Build history of the part. All positions in model axes, mm. Face numbers are marked on the shaded views. Round coordinates to 2 decimals unless told otherwise and drop trailing zeros. Write each loop counter-clockwise with the first axis right and the second up, starting at its lowest first coordinate (ties: lowest second). Pieces come first, ordered by that corner, then holes.
Item 1: Wall check: probe 1 along Z at (x, y) = (16, 0); probe 2 along X at (y, z) = (0, 21); probe 3 along Y at (x, z) = (31, -2.5). Give the ranges that are in metal, low to high.
Item 2: Band-saw the part on C-C, the plane x = -25.5. Write the cut outline in (y, z), then the cut area to 3 significant figures.
Item 3: Band-saw the part on A-A, the plane y = 0. Write the cut outline in (x, z), then the cut area to 3 significant figures.
Item 4: Drop flat-ended pins along their axis: pin 1 Ø2 at (x, y) = (-5, -19.5) entering from +Z; pin 2 Ø1 at (x, y) = (27.5, -10.5) entering from +Z; pin 3 Ø12 at (x, z) = (-11.5, -6.5) entering from -Y (3 decimals). Give the stop position or say it passes through.
Item 5: Band-saw the part on D-D, the plane y = 9.5. Write the cut outline in (x, z), then the cut area to 3 significant figures.
Item 6: Band-saw the part on B-B, the plane z = 10.5. Write the cut outline in (x, y).
Item 7: Mould opens along X. For the marked faces 1, 2, 3 and 4 say: +X half, -X half, draft (parallel to the pull), parting line (faces both ways), or undercut.
```python
from build123d import *

# Parameters (mm, degrees)
F0_R          = 25
F1_DEPTH      = 40
F2_R          = 12.5
F3_DEPTH      = 25
F4_R          = 12.5
F5_DEPTH      = 40.001
F5_DEPTH_BACK = 40.001


with BuildPart() as f1:
    # F0 (on Right) → F1 (new body, symmetric)
    with BuildSketch(Plane.YZ):
        Circle(F0_R)
    extrude(amount=F1_DEPTH, both=True)

    # F2 (on Top) → F3 (cut)
    with BuildSketch(Plane.XY):
        Circle(F2_R)
    extrude(amount=F3_DEPTH, mode=Mode.SUBTRACT)

    # F4 (on Right) → F5 (cut, two sides)
    with BuildSketch(Plane.YZ) as f5_sk:
        Circle(F4_R)
    extrude(amount=F5_DEPTH, mode=Mode.SUBTRACT)
    extrude(f5_sk.sketch, amount=-F5_DEPTH_BACK, mode=Mode.SUBTRACT)


solid = f1.part
```
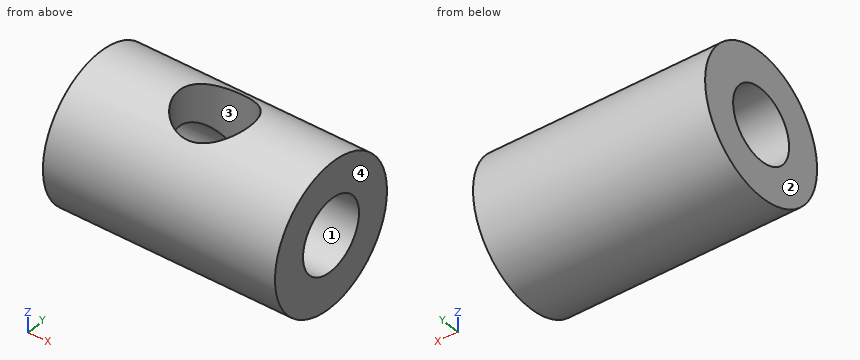
Results:
1. probe 1: z = -25 to -12.5, 12.5 to 25
1. probe 2: x = -40 to -12.5, 12.5 to 40
1. probe 3: y = -24.87 to -12.25, 12.25 to 24.87
2. outline: circle Ø50 at (0, 0); hole circle Ø25 at (0, 0)
2. area: 1,470 mm2
3. outline: (-40, -25) - (40, -25) - (40, -12.5) - (-40, -12.5) - close; (-40, 12.5) - (-12.5, 12.5) - (-12.5, 25) - (-40, 25) - close; (12.5, 12.5) - (40, 12.5) - (40, 25) - (12.5, 25) - close
3. area: 1,690 mm2
4. pin 1: stops at z = 16.82
4. pin 2: stops at z = 22.91
4. pin 3: stops at y = -24.995
5. outline: (-40, -23.12) - (40, -23.12) - (40, -8.12) - (-40, -8.12) - close; (-40, 8.12) - (-8.12, 8.12) - (-8.12, 23.12) - (-40, 23.12) - close; (8.12, 8.12) - (40, 8.12) - (40, 23.12) - (8.12, 23.12) - close
5. area: 2,160 mm2
6. outline: (-40, -22.69) - (40, -22.69) - (40, -6.78) - (10.5, -6.78) arc R12.5 cw to (-10.5, -6.78) - (-40, -6.78) - close; (-40, 6.78) - (-10.5, 6.78) arc R12.5 cw to (10.5, 6.78) - (40, 6.78) - (40, 22.69) - (-40, 22.69) - close
7. face 1: draft
7. face 2: -X half
7. face 3: undercut
7. face 4: +X half
